The model under review builds one solid part; all positions refer to its coordinate system, in mm. Face numbers are marked on the shaded views. A direction names the side the tool comes from. Give positions to 0.01 mm unless a question says otherwise; leave off trailing zeros. Loops run counter-clockwise (first coordinate to the right, second up) from the corner with the lowest first, then second, coordinate; pieces in that order, holes last. Notation, with made-up numbers: M -9,33 L 12,33 A27 cw 12,53 Z; hole C 8.5,64.5 d7. An arc over 180 degrees is marked long. Write item = value, one per line. Start each with the question number.
1. Wall thickness on line 1 along Y through (x, z) = (43.25, 0) (3 decimals); line 2 along Z through (x, y) = (48, -6); line 3 along Y through (x, z) = (48.75, 0) (3 decimals): over which ranges is each line inside the solid? List them lowest first. Write a range as from..to.
2. We need section A-A on x = -15.5. Give the boundary of the cut face in (y, z) (1 decimal).
3. We need section D-D on z = -10. Give the boundary of the cut face in (x, y) (3 decimals), then the cut area to 3 significant figures.
4. We need section B-B on y = 26.5. Give the boundary of the cut face in (x, z) (1 decimal), then the cut area to 3 significant figures.
5. For pin 1 (5 mm diameter, centred on x = 0, y = 0, fed in from +Z); pin 2 (6 mm diameter, centred on y = -6.35, z = 0, fed in from +X) (3 decimals); pin 3 (5 mm diameter, centred on x = -20.5, y = -24, fed in from -Z); pin 4 (4 mm diameter, centred on y = 9.5, z = -9.5, fed in from -X) (3 decimals), all flat-tipped, find the tip position at first contact; note any pin that passes through.
6. Draft analysis for pull direction Y (two halves, no side actions). For the marked faces 4, 5, 6 and 7, state which applies: pulls with the +Y half, pulls with the -Y half, needs draft (parallel to the pull), parting line crosses it, or undercut.
7. For the marked faces 1, 2 and 3, list the 3-axis set-ups (+Z, -Z, +X, -X, +Y, -Y) from which the entire face can be reached by the end or side of a thin tool; tool diameter is ignored.
8. We need section C-C on x = 42.5. Give the boundary of the cut face in (y, z) (3 decimals), then the cut area to 3 significant figures.
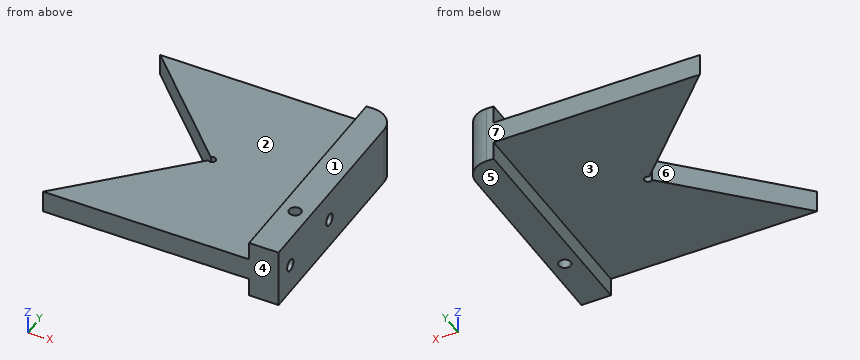
from build123d import *

# Parameters (mm, degrees)
BOSS_EXTRUDE1_DEPTH         = 4.7625
SKETCH2_R                   = 1.5875
CUT_EXTRUDE1_DEPTH          = 10.525
SKETCH3_W                   = 25.4
SKETCH3_H                   = 95.25
BOSS_EXTRUDE2_DEPTH         = 12.7
FILLET1_R                   = 9.525
F_1_4_20_TAPPED_HOLE1_D     = 5.1054
F_1_4_20_TAPPED_HOLE1_DEPTH = 15.875
F_1_4_20_TAPPED_HOLE1_TIP   = 1.533816902
F_1_4_20_TAPPED_HOLE2_D     = 5.1054


with BuildPart() as part:
    # Sketch1 → Boss-Extrude1 (new body, symmetric)
    with BuildSketch(Plane.XY):
        Polygon((-47.625, 47.625), (41.275, 47.625), (41.275, -47.625), (-47.625, -47.625), (0, 0), align=None)
    extrude(amount=BOSS_EXTRUDE1_DEPTH, both=True)

    # Sketch2 → Cut-Extrude1 (cut, through all)
    with BuildSketch(Plane.XY.offset(4.7625)):
        Circle(SKETCH2_R)
    extrude(amount=-CUT_EXTRUDE1_DEPTH, mode=Mode.SUBTRACT)

    # Sketch3 → Boss-Extrude2 (add)
    with BuildSketch(Plane(origin=(41.275, 0, 0), x_dir=(0, 0, -1), z_dir=(1, 0, 0))):
        Rectangle(SKETCH3_W, SKETCH3_H)
    extrude(amount=BOSS_EXTRUDE2_DEPTH)

    # Fillet1
    fillet1_edges = [part.edges().sort_by_distance(p)[0] for p in [
        (53.975, 47.625, 0),
    ]]
    fillet(fillet1_edges, radius=FILLET1_R)

    # 1/4-20 Tapped Hole1
    with Locations(Plane(origin=(53.975, 0, 0), x_dir=(0, 0, -1), z_dir=(1, 0, 0))):
        with Locations((0, -38.1), (0, -6.35)):
            Hole(F_1_4_20_TAPPED_HOLE1_D / 2, depth=F_1_4_20_TAPPED_HOLE1_DEPTH)
            with Locations((0, 0, -(F_1_4_20_TAPPED_HOLE1_DEPTH + F_1_4_20_TAPPED_HOLE1_TIP / 2))):  # 118° drill point
                Cone(0, F_1_4_20_TAPPED_HOLE1_D / 2, F_1_4_20_TAPPED_HOLE1_TIP, mode=Mode.SUBTRACT)

    # 1/4-20 Tapped Hole2 (through all)
    with Locations(Plane.XY.offset(12.7)):
        with Locations((47.625, -22.225)):
            Hole(F_1_4_20_TAPPED_HOLE2_D / 2)


solid = part.part
Final values:
q1.line_1 = -47.625..-40.653, -35.547..-8.903, -3.797..47.625
q1.line_2 = -12.7..-2.53, 2.53..12.7
q1.line_3 = -47.625..-40.653, -35.547..-24.516, -19.934..-8.903, -3.797..46.599
q2.outline = M -47.6,-4.8 L -15.5,-4.8 L -15.5,4.8 L -47.6,4.8 Z; M 15.5,-4.8 L 47.6,-4.8 L 47.6,4.8 L 15.5,4.8 Z
q3.outline = M 41.275,-47.625 L 53.975,-47.625 L 53.975,38.1 A9.525 ccw 44.45,47.625 L 41.275,47.625 Z; hole C 47.625,-22.225 d5.105
q3.area = 1,170 mm²
q4.outline = M -26.5,-4.8 L 41.3,-4.8 L 41.3,-12.7 L 54,-12.7 L 54,12.7 L 41.3,12.7 L 41.3,4.8 L -26.5,4.8 Z
q4.area = 968 mm²
q5.pin_1 = 4.76
q5.pin_2 = 53.975
q5.pin_3 = -4.76
q5.pin_4 = 41.275
q6.face_4 = pulls with the -Y half
q6.face_5 = needs draft
q6.face_6 = undercut
q6.face_7 = pulls with the +Y half
q7.face_1 = +Z, +X, -X, +Y, -Y
q7.face_2 = +Z, -X, +Y, -Y
q7.face_3 = -Z, -X, +Y, -Y
q8.outline = M -47.625,-12.7 L 47.625,-12.7 L 47.625,12.7 L -47.625,12.7 Z; hole C -38.1,0 d5.105; hole C -6.35,0 d5.105
q8.area = 2,380 mm²
